from build123d import *

# Parameters (mm, degrees)
F0_W     = 10
F0_H     = 85
F1_DEPTH = 3
F2_R     = 5
F4_DEPTH = 25


# Not quite as in the source:
# - a feature names something its author has since deleted; it is built from what else it names


with BuildPart() as f1:
    # F0 (on Top) → F1 (new body)
    with BuildSketch(Plane.XY):
        Polygon((45, 30), (-45, 30), (-45, 0), (-5, 0), (5, 0), (45, 0), align=None)
        with Locations((0, -42.5)):
            Rectangle(F0_W, F0_H)
    extrude(amount=F1_DEPTH)

    # F2
    f2_edges = [f1.edges().sort_by_distance(p)[0] for p in [
        (-45, 0, 1.5),
        (-45, 30, 1.5),
        (45, 0, 1.5),
        (45, 30, 1.5),
        (5, 0, 1.5),
        (-5, 0, 1.5),
    ]]
    fillet(f2_edges, radius=F2_R)

    # F3 (on face) → F4 (cut)
    with BuildSketch(Plane.XY.offset(3)):
        Polygon((-5, -85), (0, -85), (-5, -74.790418148), align=None)
        Polygon((5, -74.790418148), (0, -85), (5, -85), align=None)
    extrude(amount=-F4_DEPTH, mode=Mode.SUBTRACT)


solid = f1.part
The listing builds one solid part. Answer for the finished solid, in the listing's coordinates (mm). A direction names the side the tool comes from. Give positions to 0.01 mm unless a question says otherwise; leave off trailing zeros. Write each loop counter-clockwise with the first axis right and the second up, starting at its lowest first coordinate (ties: lowest second). Pieces come first, ordered by that corner, then holes. Notation, with made-up numbers: (55.25, 26) -> (98.25, 26) arc R22 cw to (98.25, 36) -> close; hole circle Ø9 at (80, -26). An arc over 180 degrees is marked (long way). Use a Markdown table: item, result.
(1) Flat-ended cylindrical pins translate along their axes: P1, Ø1.5, axis at x = 3.5, z = 1, coming from the -Y side; P2, Ø1.5, axis at x = 18, z = 1, coming from the -Y side; P3, Ø1.5, axis at y = -30.5, z = 1, coming from the +X side. Find the tip coordinate at first contact, or state that the pin passes through.
Return value:
| item | result |
|---|---|
| P1 | y = -79.38 |
| P2 | y = 0 |
| P3 | x = 5 |
(2) Section B-B, the plane y = 2 is taken. Determine the outline of the cut face in (x, z), then the cut area to 3 significant figures.
Return value:
| item | result |
|---|---|
| outline | (-44, 0) -> (44, 0) -> (44, 3) -> (-44, 3) -> close |
| area | 264 mm2 |
(3) Section C-C, the plane x = -25 is taken. Determine the outline of the cut face in (y, z), then the cut area to 3 significant figures.
Return value:
| item | result |
|---|---|
| outline | (0, 0) -> (30, 0) -> (30, 3) -> (0, 3) -> close |
| area | 90.0 mm2 |
(4) Section A-A, the plane z = 2 is taken. Determine the outline of the cut face in (x, y).
Return value:
| item | result |
|---|---|
| outline | (-45, 5) arc R5 ccw to (-40, 0) -> (-10, 0) arc R5 cw to (-5, -5) -> (-5, -74.79) -> (0, -85) -> (5, -74.79) -> (5, -5) arc R5 cw to (10, 0) -> (40, 0) arc R5 ccw to (45, 5) -> (45, 25) arc R5 ccw to (40, 30) -> (-40, 30) arc R5 ccw to (-45, 25) -> close |
(5) Find the intervals of material crossed by probe 1 along X at (y, z) = (-53.5, 1.3); probe 2 along Y at (x, z) = (27.5, 1.1); probe 3 along X at (y, z) = (-0.5, 2.25), in increasing order. Write a range as from..to.
Return value:
| item | result |
|---|---|
| probe 1 | -5..5 |
| probe 2 | 0..30 |
| probe 3 | -7.82..7.82 |
(6) For faces 1 (the flat face through (-5, -40, 1)), 2 (the flat face through (1, 30, 1)), 3 (the flat face through (5, -40, 1)), determine the directions among +Z, -Z, +X, -X, +Y, -Y from which every point of the face is accessible in a straight line to the end or side of a thin tool.
Return value:
| item | result |
|---|---|
| face 1 | +Z, -Z, -X, -Y |
| face 2 | +Z, -Z, +X, -X, +Y |
| face 3 | +Z, -Z, +X, -Y |
